Design review of the part built by this model. Coordinates are the model's own, in mm. A direction names the side the tool comes from. Round coordinates to 2 decimals unless told otherwise and drop trailing zeros. Write each loop counter-clockwise with the first axis right and the second up, starting at its lowest first coordinate (ties: lowest second). Pieces come first, ordered by that corner, then holes.
from build123d import *

# Parameters (mm, degrees)
F0_W     = 450
F0_H     = 450
F0_R     = 23.781071
F1_DEPTH = 40
F2_R     = 23.781071
F3_DEPTH = 420
F4_R     = 10
F5_R     = 10


with BuildPart() as f1:
    # F0 (on Top) → F1 (new body)
    with BuildSketch(Plane.XY):
        Rectangle(F0_W, F0_H)
        with Locations((-200, -200)):
            Circle(F0_R, mode=Mode.SUBTRACT)
        with Locations((200, -200)):
            Circle(F0_R, mode=Mode.SUBTRACT)
        with Locations((-200, 200)):
            Circle(F0_R, mode=Mode.SUBTRACT)
        with Locations((200, 200)):
            Circle(F0_R, mode=Mode.SUBTRACT)
    extrude(amount=F1_DEPTH)

    # F2 (on face) → F3 (join)
    with BuildSketch(Plane.XY.offset(40)):
        with Locations((-200, -200)):
            Circle(F2_R)
        with Locations((-200, 200)):
            Circle(F2_R)
        with Locations((200, 200)):
            Circle(F2_R)
        with Locations((200, -200)):
            Circle(F2_R)
    extrude(amount=-F3_DEPTH)

    # F4
    f4_edges = [f1.edges().sort_by_distance(p)[0] for p in [
        (-223.781071, -200, -380),
        (176.218929, -200, -380),
        (176.218929, 200, -380),
        (-223.781071, 200, -380),
    ]]
    fillet(f4_edges, radius=F4_R)

    # F5
    f5_edges = [f1.edges().sort_by_distance(p)[0] for p in [
        (225, -225, 20),
        (225, 225, 20),
        (-225, -225, 20),
        (-225, 225, 20),
    ]]
    fillet(f5_edges, radius=F5_R)


solid = f1.part
1) For P1, Ø3, axis at x = -107.5, y = 131.5, coming from the -Z side; P2, Ø10, axis at y = 125.5, z = -8.5, coming from the -X side, all flat-tipped, find the tip position at first contact; note any pin that passes through.
2) Add section D-D on x = -137. State the section outline as (y, z) points, and give its area (3 significant figures).
3) Add section A-A on x = 200. State the section outline as (y, z) points, and give its area (3 significant figures).
4) Add section B-B on z = -50.5. State the section outline as (x, y) points.
5) For line 1 along Y through (x, z) = (201.5, -175); line 2 along Z through (x, y) = (81.5, 102); line 3 along X through (y, z) = (185.5, -86.5), list the stretches that pass through material, from the lowest coordinate up.
6) For faces 1 (the face through (-205.155, -223.216, -182.41)), 2 (the face through (-225, -3, 20)), list the 3-axis set-ups (+Z, -Z, +X, -X, +Y, -Y) from which the entire face can be reached by the end or side of a thin tool; tool diameter is ignored.
7) The part is to be moulded in two halves that separate along Y. For faces 3 (the face through (-3, 225, 20)), 4 (the face through (-205.155, 176.784, -182.41)), 5 (the face through (194.845, -223.216, -182.41)), 6 (the face through (225, -3, 20)), say which applies: pulls with the +Y half, pulls with the -Y half, needs draft (parallel to the pull), parting line crosses it, or undercut.
Computed:
1. P1: stops at z = 0
1. P2: passes through
2. outline: (-225, 0) - (225, 0) - (225, 40) - (-225, 40) - close
2. area: 18,000 mm2
3. outline: (-225, 0) - (-223.78, 0) - (-223.78, -370) arc R10 ccw to (-213.78, -380) - (-186.22, -380) arc R10 ccw to (-176.22, -370) - (-176.22, 0) - (176.22, 0) - (176.22, -370) arc R10 ccw to (186.22, -380) - (213.78, -380) arc R10 ccw to (223.78, -370) - (223.78, 0) - (225, 0) - (225, 40) - (-225, 40) - close
3. area: 54,100 mm2
4. outline: circle Ø47.56 at (-200, -200); circle Ø47.56 at (-200, 200); circle Ø47.56 at (200, -200); circle Ø47.56 at (200, 200)
5. line 1: y = -223.73 to -176.27, 176.27 to 223.73
5. line 2: z = 0 to 40
5. line 3: x = -218.85 to -181.15, 181.15 to 218.85
6. face 1: -Z
6. face 2: +Z, -Z, -X, +Y, -Y
7. face 3: pulls with the +Y half
7. face 4: undercut
7. face 5: undercut
7. face 6: needs draft
